```python
from build123d import *

# Parameters (mm, degrees)
F0_W     = 138.5640646055
F0_H     = 20
F1_DEPTH = 3.175
F3_DEPTH = 3.175


# Not quite as in the source:
# - a length typed as a fraction of an inch, garbled in the dataset ("3 / 203.2 mm" for 3/8 in), is restored


with BuildPart() as f1:
    # F0 (on Top) → F1 (new body)
    with BuildSketch(Plane.XY):
        with BuildLine():
            Line((77.9422863406, -35), (21.6506350946, 62.5))
            ThreePointArc((21.6506350946, 62.5), (0, 75), (-21.6506350946, 62.5))
            Line((-21.6506350946, 62.5), (-77.9422863406, -35))
            ThreePointArc((-77.9422863406, -35), (-77.9422863406, -45), (-69.2820323028, -50))
            Line((-69.2820323028, -50), (69.2820323028, -50))
            ThreePointArc((69.2820323028, -50), (77.9422863406, -45), (77.9422863406, -35))
        make_face()
        with Locations((0, -60)):
            Rectangle(F0_W, F0_H)
    extrude(amount=F1_DEPTH)

    # F2 (on face) → F3 (cut, through all)
    with BuildSketch(Plane.XY.offset(3.175)):
        with BuildLine():
            ThreePointArc((2.4179291552, 34.2129931944), (7.5417637262, 30.8178539771), (9.525, 25))
            ThreePointArc((9.525, 25), (5.8178542624, 17.4582364939), (-2.4179284582, 15.7870066226))
            Line((-2.4179284582, 15.7870066226), (57.735026919, 0))
            Line((57.735026919, 0), (44.3333494626, 23.2123862611))
            Line((44.3333494626, 23.2123862611), (2.4179291552, 34.2129931944))
        make_face()
        with BuildLine():
            ThreePointArc((-2.4179284582, 15.7870066226), (5.8178542624, 17.4582364939), (9.525, 25))
            ThreePointArc((9.525, 25), (7.5417637262, 30.8178539771), (2.4179291552, 34.2129931944))
            ThreePointArc((2.4179291552, 34.2129931944), (-9.2129932859, 27.4179288067), (-2.4179284582, 15.7870066226))
        make_face()
    extrude(amount=-F3_DEPTH, mode=Mode.SUBTRACT)


solid = f1.part
```
Geometry: final body of the model. Coordinates: model frame, mm. A direction names the side the tool comes from. Coordinates: 2 decimals unless noted, no trailing zeros. Order: outer loops, then holes, each group sorted by start corner. A loop starts at its lowest first (then second) coordinate and runs counter-clockwise, first axis right, second up. Notation, with made-up numbers: (33, 63.5) -> (61, 63.5) arc R15 cw to (61, 79.5) -> close; hole circle Ø6 at (4.25, -5.75). An arc over 180 degrees is marked (long way). Write item = value, one per line.
(1) Line query: line 1 (Y direction, x = 33, z = 1.65); line 2 (Y direction, x = 44, z = 1.6); line 3 (X direction, y = -40.5, z = 2.1). Output: solid intervals per line, ascending.
Solved:
line_1 = -70 to 6.49, 26.19 to 42.84
line_2 = -70 to 3.6, 23.3 to 23.79
line_3 = -79.27 to 79.27
(2) Cut plane D-D on x = -41. Return loops of the section in (y, z) (3 decimals).
Solved:
outline = (-70, 0) -> (28.986, 0) -> (28.986, 3.175) -> (-70, 3.175) -> close
(3) Cut plane C-C on y = -7.5. Return loops of the section in (x, z) (3 decimals), plus the area to 3 significant figures.
Solved:
outline = (-62.065, 0) -> (62.065, 0) -> (62.065, 3.175) -> (-62.065, 3.175) -> close
area = 394 mm²
(4) Pin query (flat end, axial travel): pin 1 Ø1.5 at (y, z) = (60, 0.5) entering from +X; pin 2 Ø1.5 at (x, z) = (23.5, 2.5) entering from +Y; pin 3 Ø1.6 at (y, z) = (-63.5, 2) entering from -X. Return the tip coordinate at first contact, or that it passes through.
Solved:
pin_1 = 23.53
pin_2 = 60.6
pin_3 = -69.28
(5) Cut plane B-B on y = 25. Return loops of the section in (x, z) (3 decimals).
Solved:
outline = (-43.301, 0) -> (-9.525, 0) -> (-9.525, 3.175) -> (-43.301, 3.175) -> close; (37.522, 0) -> (43.301, 0) -> (43.301, 3.175) -> (37.522, 3.175) -> close
(6) Cut plane A-A on x = 0. Return loops of the section in (y, z) (3 decimals), plus the area to 3 significant figures.
Solved:
outline = (-70, 0) -> (15.152, 0) -> (15.152, 3.175) -> (-70, 3.175) -> close; (34.525, 0) -> (75, 0) -> (75, 3.175) -> (34.525, 3.175) -> close
area = 399 mm²
(7) Access query for faces 1 (the flat face through (27.237, 8.004, 1.61)), 2 (the flat face through (67.98, -17.745, 1.565)). Directions: +Z, -Z, +X, -X, +Y, -Y. A direction counts if a zero-diameter tool reaches every point of the face in a straight line with its end or side. Return the directions, or none.
Solved:
face_1 = +Z, -Z, +X
face_2 = +Z, -Z, +X, +Y
(8) Pull-direction query (X, two-part tool) for faces 3 (the flat face through (-49.402, 14.432, 1.565)), 4 (the flat face through (23.669, 28.636, 1.61)), 5 (the cylindrical face through (0, 75, 2)); classes: pulls with the +X half, pulls with the -X half, needs draft (parallel to the pull), parting line crosses it, or undercut.
Solved:
face_3 = pulls with the -X half
face_4 = undercut
face_5 = parting line crosses it
